Input: dimensioned drawing with shaded views. Units: mm. Origin: part minimum x, y, z. Coordinates: 2 decimals unless noted, no trailing zeros. Write each loop counter-clockwise with the first axis right and the second up, starting at its lowest first coordinate (ties: lowest second). Pieces come first, ordered by that corner, then holes. Notation, with made-up numbers: (20.5, 13.5) -> (60.5, 13.5) arc R15 ccw to (60.5, 39.5) -> close; hole circle Ø6 at (76.5, 21). An arc over 180 degrees is marked (long way). One line per item, written item: value. Start each with the question number.
1. Section query A-A, the plane x = 15. State how many separate pieces and enclosed holes the cut face has, and give its area (3 significant figures).
2. First-contact query: P1, Ø2, axis at y = 29.5, z = 13.5, coming from the +X side; P2, Ø1, axis at x = 6, z = 9, coming from the +Y side (1 decimal); P3, Ø2, axis at x = 13.5, y = 4, coming from the -Z side. Flat tips, straight axial feed; report the tip coordinate or a pass-through.
3. Section query D-D, the plane y = 42.5. Output: boundary loops of the cut face in (x, z).
4. Line query: line 1 (Y direction, x = 15, z = 8); line 2 (Y direction, x = 15, z = 27.4) (1 decimal); line 3 (Y direction, x = 24, z = 3.5). Output: solid intervals per line, ascending.
5. Section query B-B, the plane z = 7. Output: boundary loops of the cut face in (x, y) (1 decimal).
6. Section query C-C, the plane z = 15. Output: boundary loops of the cut face in (x, y), and give its area (3 significant figures).
7. Mould query, pull axis Z, two halves, no side actions, for the marked faces 1, 2 and 3. Classes: released by +Z, released by -Z, zero draft, split by the parting line, or undercut.
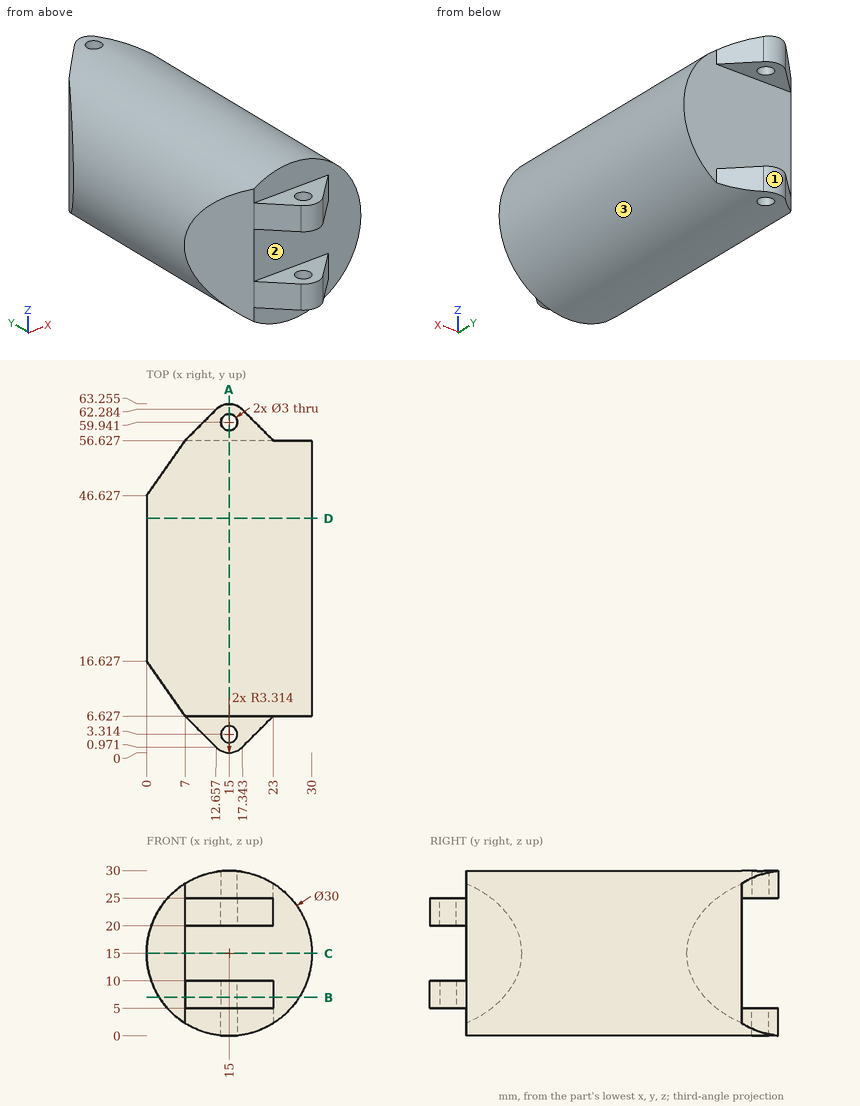
Computed values:
1. separate pieces: 5
1. enclosed holes: 0
1. area: 1,570 mm²
2. P1: stops at x = 29.99
2. P2: stops at y = 55.9
2. P3: stops at z = 5
3. outline: circle Ø30 at (15, 15)
4. line 1: y = 0 to 1.81, 4.81 to 56.63
4. line 2: y = 6.6 to 58.4, 61.4 to 63.3
4. line 3: y = 6.63 to 56.63
5. outline: (2.3, 13.3) -> (7, 6.6) -> (12.7, 1) arc R3.3 ccw to (17.3, 1) -> (23, 6.6) -> (27.7, 6.6) -> (27.7, 56.6) -> (7, 56.6) -> (2.3, 49.9) -> close; hole circle Ø3 at (15, 3.3)
6. outline: (0, 16.63) -> (7, 6.63) -> (30, 6.63) -> (30, 56.63) -> (7, 56.63) -> (0, 46.63) -> close
6. area: 1,430 mm²
7. face 1: zero draft
7. face 2: undercut
7. face 3: split by the parting line
